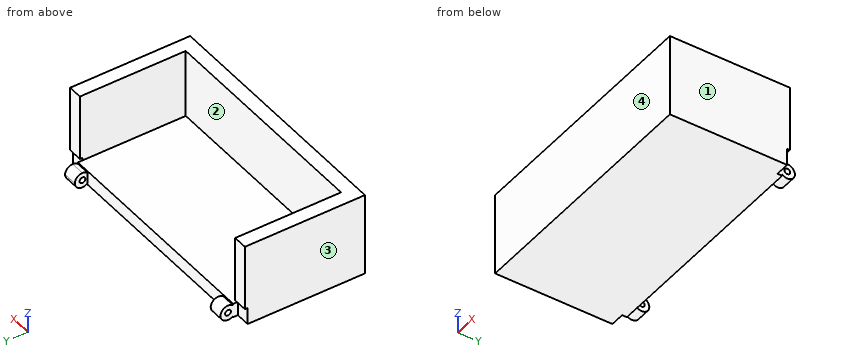
```python
from build123d import *

# Parameters (mm, degrees)
SKETCH1_W            = 269.8
SKETCH1_H            = 142.5
BOSS_EXTRUDE2_DEPTH  = 15
SKETCH2_W            = 239.8
SKETCH2_H            = 112.5
CUT_EXTRUDE1_DEPTH   = 5
BOSS_EXTRUDE3_DEPTH  = 75
SKETCH7_R            = 8.089056034
SKETCH7_R_2          = 3.089056034
BOSS_EXTRUDE4_DEPTH  = 15
BOSS_EXTRUDE5_DEPTH  = 15
SKETCH15_W           = 15
SKETCH15_H           = 15
CUT_EXTRUDE2_DEPTH   = 5
SKETCH16_W           = 269.8
SKETCH16_H           = 127.5
CUT_EXTRUDE3_DEPTH   = 49
SKETCH17_W           = 269.8
SKETCH17_H           = 15
BOSS_EXTRUDE6_DEPTH  = 39.6
BOSS_EXTRUDE8_DEPTH  = 72.95
SKETCH20_W           = 15
SKETCH20_H           = 70.089840249
BOSS_EXTRUDE9_DEPTH  = 2.85
SKETCH21_W           = 15
SKETCH21_H           = 70.0898402
BOSS_EXTRUDE10_DEPTH = 2.85


with BuildPart() as part:
    # Sketch1 → Boss-Extrude2 (new body)
    with BuildSketch(Plane(origin=(0, 0, 0), x_dir=(1, 0, 0), z_dir=(0, 1, 0))):
        with Locations((-23.308401977, 12.292504119)):
            Rectangle(SKETCH1_W, SKETCH1_H)
    extrude(amount=BOSS_EXTRUDE2_DEPTH)

    # Sketch2 → Cut-Extrude1 (cut)
    with BuildSketch(Plane(origin=(0, 15, 0), x_dir=(1, 0, 0), z_dir=(0, 1, 0))):
        with Locations((-23.308401977, 12.292504119)):
            Rectangle(SKETCH2_W, SKETCH2_H)
    extrude(amount=-CUT_EXTRUDE1_DEPTH, mode=Mode.SUBTRACT)

    # Sketch3 → Boss-Extrude3 (add)
    with BuildSketch(Plane(origin=(0, 15, 0), x_dir=(1, 0, 0), z_dir=(0, 1, 0))):
        Polygon((-143.208401977, 68.542504119), (-158.208401977, 68.542504119), (-158.208401977, 83.542504119), (111.591598023, 83.542504119), (111.591598023, 68.542504119), align=None)
    extrude(amount=BOSS_EXTRUDE3_DEPTH)

    # Sketch7 → Boss-Extrude4 (add)
    with BuildSketch(Plane(origin=(-143.208401977, 0, 0), x_dir=(0, 0, -1), z_dir=(1, 0, 0))):
        with Locations((76.070987498, 95.45383679)):
            Circle(SKETCH7_R)
        with Locations((76.070987498, 95.45383679)):
            Circle(SKETCH7_R_2, mode=Mode.SUBTRACT)
    extrude(amount=BOSS_EXTRUDE4_DEPTH)

    # Sketch12 → Boss-Extrude5 (add)
    with BuildSketch(Plane.ZY.offset(-96.591598023)):
        with BuildLine():
            ThreePointArc((-76.070987498, 103.542892824), (-84.160043532, 95.45383679), (-76.070987498, 87.364780756))
            Line((-76.070987498, 87.364780756), (-76.070987498, 92.364780756))
            ThreePointArc((-76.070987498, 92.364780756), (-79.160043532, 95.45383679), (-76.070987498, 98.542892824))
            Line((-76.070987498, 98.542892824), (-76.070987498, 103.542892824))
        make_face()
        with BuildLine():
            Line((-76.070987498, 92.364780756), (-76.070987498, 87.364780756))
            ThreePointArc((-76.070987498, 87.364780756), (-70.351161122, 89.734010415), (-67.981931463, 95.45383679))
            ThreePointArc((-67.981931463, 95.45383679), (-70.351161122, 101.173663165), (-76.070987498, 103.542892824))
            Line((-76.070987498, 103.542892824), (-76.070987498, 98.542892824))
            ThreePointArc((-76.070987498, 98.542892824), (-73.886695028, 97.638129259), (-72.981931463, 95.45383679))
            ThreePointArc((-72.981931463, 95.45383679), (-73.886695028, 93.269544321), (-76.070987498, 92.364780756))
        make_face()
    extrude(amount=BOSS_EXTRUDE5_DEPTH)

    # Sketch15 → Cut-Extrude2 (cut)
    with BuildSketch(Plane(origin=(0, 90, 0), x_dir=(1, 0, 0), z_dir=(0, 1, 0))):
        with Locations((-150.708401977, 76.042504119)):
            Rectangle(SKETCH15_W, SKETCH15_H)
        with Locations((104.091598023, 76.042504119)):
            Rectangle(SKETCH15_W, SKETCH15_H)
    extrude(amount=-CUT_EXTRUDE2_DEPTH, mode=Mode.SUBTRACT)

    # Sketch16 → Cut-Extrude3 (cut)
    with BuildSketch(Plane(origin=(0, 25, 0), x_dir=(1, 0, 0), z_dir=(0, 1, 0))):
        with Locations((-23.308401977, 4.792504119)):
            Rectangle(SKETCH16_W, SKETCH16_H)
    extrude(amount=-CUT_EXTRUDE3_DEPTH, mode=Mode.SUBTRACT)

    # Sketch17 → Boss-Extrude6 (add)
    with BuildSketch(Plane.XZ):
        with Locations((-23.308401977, -76.042504119)):
            Rectangle(SKETCH17_W, SKETCH17_H)
    extrude(amount=BOSS_EXTRUDE6_DEPTH)

    # Sketch19 → Boss-Extrude8 (add)
    with BuildSketch(Plane.XY.offset(-68.542504119)):
        Polygon((-158.208401977, 85), (-158.208401977, -39.6), (111.591598023, -39.6), (111.591598023, 85), (96.591598023, 85), (96.591598023, -24.6), (-143.208401977, -24.6), (-143.208401977, 85), align=None)
    extrude(amount=BOSS_EXTRUDE8_DEPTH)

    # Sketch20 → Boss-Extrude9 (add)
    with BuildSketch(Plane(origin=(0, 85, 0), x_dir=(1, 0, 0), z_dir=(0, 1, 0))):
        with Locations((-150.708401977, 30.637424243)):
            Rectangle(SKETCH20_W, SKETCH20_H)
    extrude(amount=BOSS_EXTRUDE9_DEPTH)

    # Sketch21 → Boss-Extrude10 (add)
    with BuildSketch(Plane(origin=(0, 85, 0), x_dir=(1, 0, 0), z_dir=(0, 1, 0))):
        with Locations((104.091598023, 30.637424219)):
            Rectangle(SKETCH21_W, SKETCH21_H)
    extrude(amount=BOSS_EXTRUDE10_DEPTH)


solid = part.part
```
Check sheet for the modelled part. Datum: model origin and axes. Units: mm. Face numbers are marked on the shaded views. Coordinates: 2 decimals unless noted, no trailing zeros. Loops run counter-clockwise (first coordinate to the right, second up) from the corner with the lowest first, then second, coordinate; pieces in that order, holes last.
1) Material ranges on probe 1 along X at (y, z) = (-3.5, -32.5); probe 2 along Y at (x, z) = (90, -76.5); probe 3 along Y at (x, z) = (72, -19), recorded low to high.
2) Release check for a two-part mould opening along X. For the marked faces 1, 2, 3 and 4 record: released by +X, released by -X, zero draft, split by the parting line, or undercut.
3) Gauge pin test, flat ends, axial feed: pin 1 (8 mm diameter, centred on x = 35, y = 85.5, fed in from +Z); pin 2 (2.5 mm diameter, centred on x = 107, y = 86, fed in from -Z); pin 3 (7.5 mm diameter, centred on x = -153, z = -27, fed in from +Y). Record the tip position at first contact, or that the pin passes through.
4) Sectioned sample at A-A (z = -27). Record the boundary of the cut face in (x, y), and give its area (3 significant figures).
5) Sectioned sample at B-B (x = -103). Record the boundary of the cut face in (y, z).
6) Sectioned sample at C-C (y = 40). Record the boundary of the cut face in (x, z).
Check sheet entries:
1. probe 1: x = -158.21 to -143.21, 96.59 to 111.59
1. probe 2: y = -39.6 to 92.39, 98.51 to 103.53
1. probe 3: y = -39.6 to -24.6
2. face 1: released by +X
2. face 2: undercut
2. face 3: released by -X
2. face 4: zero draft
3. pin 1: stops at z = -68.54
3. pin 2: stops at z = -83.54
3. pin 3: stops at y = 87.85
4. outline: (-158.21, -39.6) - (111.59, -39.6) - (111.59, 87.85) - (96.59, 87.85) - (96.59, -24.6) - (-143.21, -24.6) - (-143.21, 87.85) - (-158.21, 87.85) - close
4. area: 7,420 mm2
5. outline: (-39.6, -83.54) - (90, -83.54) - (90, -68.54) - (-24.6, -68.54) - (-24.6, 4.41) - (-39.6, 4.41) - close
6. outline: (-158.21, -83.54) - (111.59, -83.54) - (111.59, 4.41) - (96.59, 4.41) - (96.59, -68.54) - (-143.21, -68.54) - (-143.21, 4.41) - (-158.21, 4.41) - close
